from build123d import *

# Parameters (mm, degrees)
ESQUISSE1_R             = 6.1
ESQUISSE1_R_2           = 4
BOSS_EXTRU_1_DEPTH      = 10
ESQUISSE4_W             = 0.6
ESQUISSE4_H             = 0.3
ENL_V_MAT_EXTRU_3_DEPTH = 10


with BuildPart() as part:
    # Esquisse1 → Boss.-Extru.1 (new body)
    with BuildSketch(Plane.XY):
        Circle(ESQUISSE1_R)
        Circle(ESQUISSE1_R_2, mode=Mode.SUBTRACT)
    extrude(amount=BOSS_EXTRU_1_DEPTH)

    # Esquisse4 → Enlèv. mat.-Extru.3 (cut)
    with BuildSketch(Plane.XY.offset(10)):
        Polygon((0.767234647, 5.907948121), (0.820801716, 6.203126997), (1.411159469, 6.09599286), (1.357592401, 5.800813984), align=None)
        with Locations((0, 6.1)):
            Rectangle(ESQUISSE4_W, ESQUISSE4_H)
        Polygon((1.809809742, 5.676009928), (1.915222189, 5.956880389), (2.476963112, 5.746055494), (2.371550664, 5.465185033), align=None)
        Polygon((2.794216062, 5.261640105), (2.948085846, 5.519174743), (3.463155122, 5.211435177), (3.309285339, 4.953900539), align=None)
        Polygon((3.68881398, 4.678156841), (3.886195597, 4.90407828), (4.338038477, 4.509315045), (4.140656859, 4.283393605), align=None)
        Polygon((4.46485038, 3.944313766), (4.699399825, 4.131360706), (5.073493706, 3.662261817), (4.838944261, 3.475214876), align=None)
        Polygon((5.097382816, 3.083697201), (5.361561475, 3.2258578), (5.645882673, 2.697500481), (5.381704013, 2.555339882), align=None)
        Polygon((5.566081174, 2.123968071), (5.851398129, 2.21667317), (6.036808325, 1.64603926), (5.75149137, 1.553334162), align=None)
        Polygon((5.855881103, 1.09597286), (6.153166031, 1.13624284), (6.233705991, 0.541672983), (5.936421062, 0.501403003), align=None)
        Polygon((5.957468195, 0.032752179), (6.257166115, 0.01929273), (6.230247217, -0.58010311), (5.930549297, -0.566643661), align=None)
        Polygon((5.867577358, -1.031521183), (6.160055731, -1.098277464), (6.026543171, -1.683234211), (5.734064797, -1.616477931), align=None)
        Polygon((5.589097756, -2.062640607), (5.864956088, -2.180548116), (5.629141069, -2.73226478), (5.353282737, -2.61435727), align=None)
        Polygon((5.130979954, -3.027465064), (5.38135193, -3.192734158), (5.050813741, -3.69347811), (4.800441765, -3.528209016), align=None)
        Polygon((4.507948234, -3.894984302), (4.724786694, -4.102303097), (4.310149104, -4.535980015), (4.093310645, -4.328661221), align=None)
        Polygon((3.740027349, -4.637315541), (3.916362925, -4.880020639), (3.430952729, -5.232691791), (3.254617153, -4.989986692), align=None)
        Polygon((2.851898908, -5.230599642), (2.98206403, -5.500890303), (2.441482709, -5.761220546), (2.311317587, -5.490929886), align=None)
        Polygon((1.872108089, -5.655767967), (1.951919143, -5.944956826), (1.373541427, -6.104578933), (1.293730373, -5.815390075), align=None)
        Polygon((0.832146176, -5.899155257), (0.859037969, -6.197947545), (0.261453392, -6.25173113), (0.2345616, -5.952938842), align=None)
        Polygon((-0.2345616, -5.952938842), (-0.261453392, -6.25173113), (-0.859037969, -6.197947545), (-0.832146176, -5.899155257), align=None)
        Polygon((-1.293730373, -5.815390075), (-1.373541427, -6.104578933), (-1.951919143, -5.944956826), (-1.872108089, -5.655767967), align=None)
        Polygon((-2.311317587, -5.490929886), (-2.441482709, -5.761220546), (-2.98206403, -5.500890303), (-2.851898908, -5.230599642), align=None)
        Polygon((-3.254617153, -4.989986692), (-3.430952729, -5.232691791), (-3.916362925, -4.880020639), (-3.740027349, -4.637315541), align=None)
        Polygon((-4.093310645, -4.328661221), (-4.310149104, -4.535980015), (-4.724786694, -4.102303097), (-4.507948234, -3.894984302), align=None)
        Polygon((-4.800441765, -3.528209016), (-5.050813741, -3.69347811), (-5.38135193, -3.192734158), (-5.130979954, -3.027465064), align=None)
        Polygon((-5.353282737, -2.61435727), (-5.629141069, -2.73226478), (-5.864956088, -2.180548116), (-5.589097756, -2.062640607), align=None)
        Polygon((-5.734064797, -1.616477931), (-6.026543171, -1.683234211), (-6.160055731, -1.098277464), (-5.867577358, -1.031521183), align=None)
        Polygon((-5.930549297, -0.566643661), (-6.230247217, -0.58010311), (-6.257166115, 0.01929273), (-5.957468195, 0.032752179), align=None)
        Polygon((-5.936421062, 0.501403003), (-6.233705991, 0.541672983), (-6.153166031, 1.13624284), (-5.855881103, 1.09597286), align=None)
        Polygon((-5.75149137, 1.553334162), (-6.036808325, 1.64603926), (-5.851398129, 2.21667317), (-5.566081174, 2.123968071), align=None)
        Polygon((-5.381704013, 2.555339882), (-5.645882673, 2.697500481), (-5.361561475, 3.2258578), (-5.097382816, 3.083697201), align=None)
        Polygon((-4.838944261, 3.475214876), (-5.073493706, 3.662261817), (-4.699399825, 4.131360706), (-4.46485038, 3.944313766), align=None)
        Polygon((-4.140656859, 4.283393605), (-4.338038477, 4.509315045), (-3.886195597, 4.90407828), (-3.68881398, 4.678156841), align=None)
        Polygon((-3.309285339, 4.953900539), (-3.463155122, 5.211435177), (-2.948085846, 5.519174743), (-2.794216062, 5.261640105), align=None)
        Polygon((-2.371550664, 5.465185033), (-2.476963112, 5.746055494), (-1.915222189, 5.956880389), (-1.809809742, 5.676009928), align=None)
        Polygon((-1.357592401, 5.800813984), (-1.411159469, 6.09599286), (-0.820801716, 6.203126997), (-0.767234647, 5.907948121), align=None)
    extrude(amount=-ENL_V_MAT_EXTRU_3_DEPTH, mode=Mode.SUBTRACT)


solid = part.part
Geometry check sheet. Reference: the model listing, model coordinates, mm. Round coordinates to 2 decimals unless told otherwise and drop trailing zeros. Loops run counter-clockwise (first coordinate to the right, second up) from the corner with the lowest first, then second, coordinate; pieces in that order, holes last. Notation, with made-up numbers: (32.5, -36.75) - (73.5, -36.75) arc R38 ccw to (73.5, 1.25) - close; hole circle Ø11 at (-38.75, 48). An arc over 180 degrees is marked (long way). One line per question, with ' | ' between items. Start each with the question number.
1. Draft check along X on faces 1 (the face through (-0.09, 4.15, 0)), 2 (the face through (-0.867, -3.905, 4.93)). Enter one of: released by +X, released by -X, zero draft, split by the parting line, or undercut.
2. Scan lines: line 1 (Y direction, x = 0, z = 5.75); line 2 (Y direction, x = -1.5, z = 8.75); line 3 (X direction, y = 2.25, z = 8.25). Record each from-to range of solid material in increasing order. Write a range as [from, to].
3. Depth check by flat-ended pin: pin 1 (1.5 mm diameter, centred on y = 1.5, z = 5, fed in from +X); pin 2 (6 mm diameter, centred on x = 4, z = 2, fed in from -Y); pin 3 (5 mm diameter, centred on x = 0, y = 0, fed in from +Z); pin 4 (2 mm diameter, centred on x = 3, z = 1, fed in from +Y). Enter the tip coordinate at first touch or a pass-through.
4. Cross-section at A-A on x = 0. Record the cut outline in (y, z), then the cut area to 3 significant figures.
Taken from the geometry:
1) face 1: zero draft | face 2: undercut
2) line 1: [-6.1, -4], [4, 5.95] | line 2: [-5.76, -3.71], [3.71, 5.91] | line 3: [-5.67, -3.31], [3.31, 5.67]
3) pin 1: x = 6 | pin 2: y = -6.02 | pin 3: through | pin 4: y = 5.6
4) outline: (-6.1, 0) - (-4, 0) - (-4, 10) - (-6.1, 10) - close; (4, 0) - (5.95, 0) - (5.95, 10) - (4, 10) - close | area: 40.5 mm²
